Can you work these out from the model? Positions are in its coordinate system, mm. Face numbers are marked on the shaded views. A direction names the side the tool comes from. Give positions to 0.01 mm unless a question says otherwise; leave off trailing zeros. Order: outer loops, then holes, each group sorted by start corner. A loop starts at its lowest first (then second) coordinate and runs counter-clockwise, first axis right, second up. Notation, with made-up numbers: M -21.5,54.25 L -14.5,54.25 A23 cw -14.5,73.25 Z; hole C 45.25,-16 d4. An arc over 180 degrees is marked long. Write each question's results on one line, items separated by ' | '.
from build123d import *

# Parameters (mm, degrees)
ESQUISSE2_W                  = 56.5
ESQUISSE2_H                  = 38
ESQUISSE2_R                  = 3.05
ESQUISSE2_W_2                = 6
SOCLESYRINGE_DEPTH           = 12
ESQUISSE2_2_R                = 3.05
BOSS_EXTRU_2_DEPTH           = 3
ESQUISSE2_4_W                = 6
ESQUISSE2_4_H                = 38
BOSS_EXTRU_4_DEPTH           = 14
ESQUISSE3_W                  = 68.5
ESQUISSE3_H                  = 20
BOSS_EXTRU_3_DEPTH           = 12
ESQUISSE4_W                  = 11
ESQUISSE4_H                  = 5.5
ENL_V_MAT_EXTRU_1_DEPTH      = 10
CONG_1_R                     = 2.7
ESQUISSE6_W                  = 68.5
ESQUISSE6_H                  = 25
BOSS_EXTRU_5_DEPTH           = 15.5
BOSS_EXTRU_6_DEPTH           = 3.6
ENL_V_MAT_EXTRU_3_DEPTH      = 80.515611675
CONG_2_R                     = 1
ENL_V_MAT_EXTRU_2_DEPTH      = 76.059126694
ENL_V_MAT_EXTRU_2_DEPTH_BACK = 76.059126694
ESQUISSE5_R                  = 2.5
ESQUISSE9_R                  = 5.5
ENL_V_MAT_EXTRU_4_DEPTH      = 24


with BuildPart() as part:
    # Esquisse2 → SocleSyringe (new body)
    # profile 1 of 3: a face of its own
    with BuildSketch(Plane.XY):
        Rectangle(ESQUISSE2_W, ESQUISSE2_H)
        with Locations((-21.5, 9)):
            Circle(ESQUISSE2_R, mode=Mode.SUBTRACT)
        with Locations((21.5, 9)):
            Circle(ESQUISSE2_R, mode=Mode.SUBTRACT)
    # profile 2 of 3: a face of its own
    with BuildSketch(Plane.XY):
        with Locations((-31.25, 0)):
            Rectangle(ESQUISSE2_W_2, ESQUISSE2_H)
    # profile 3 of 3: a face of its own
    with BuildSketch(Plane.XY):
        with Locations((31.25, 0)):
            Rectangle(ESQUISSE2_W_2, ESQUISSE2_H)
    extrude(amount=SOCLESYRINGE_DEPTH)

    # Esquisse2<2> → Boss.-Extru.2 (add)
    with BuildSketch(Plane.XY):
        with Locations((-21.5, 9)):
            Circle(ESQUISSE2_2_R)
        with Locations((21.5, 9)):
            Circle(ESQUISSE2_2_R)
    extrude(amount=BOSS_EXTRU_2_DEPTH)

    # Esquisse2<4> → Boss.-Extru.4 (add)
    with BuildSketch(Plane.XY):
        with Locations((-31.25, 0)):
            Rectangle(ESQUISSE2_4_W, ESQUISSE2_4_H)
        with Locations((31.25, 0)):
            Rectangle(ESQUISSE2_4_W, ESQUISSE2_4_H)
    extrude(amount=BOSS_EXTRU_4_DEPTH)

    # Esquisse3 → Boss.-Extru.3 (add)
    with BuildSketch(Plane.XY):
        with Locations((0, 29)):
            Rectangle(ESQUISSE3_W, ESQUISSE3_H)
    extrude(amount=BOSS_EXTRU_3_DEPTH)

    # Esquisse4 → Enlèv. mat.-Extru.1 (cut)
    with BuildSketch(Plane.XY.offset(12)):
        with Locations((-23.75, 34)):
            Rectangle(ESQUISSE4_W, ESQUISSE4_H)
        with Locations((23.75, 34)):
            Rectangle(ESQUISSE4_W, ESQUISSE4_H)
        with Locations((23.75, 24)):
            Rectangle(ESQUISSE4_W, ESQUISSE4_H)
        with Locations((-23.75, 24)):
            Rectangle(ESQUISSE4_W, ESQUISSE4_H)
        with Locations((0, 34)):
            Rectangle(ESQUISSE4_W, ESQUISSE4_H)
        with Locations((0, 24)):
            Rectangle(ESQUISSE4_W, ESQUISSE4_H)
    extrude(amount=-ENL_V_MAT_EXTRU_1_DEPTH, mode=Mode.SUBTRACT)

    # Congé1
    cong_1_edges = [part.edges().sort_by_distance(p)[0] for p in [
        (23.75, 36.75, 2),
        (23.75, 31.25, 2),
        (23.75, 26.75, 2),
        (23.75, 21.25, 2),
        (-23.75, 21.25, 2),
        (-23.75, 26.75, 2),
        (0, 31.25, 2),
        (0, 36.75, 2),
        (0, 21.25, 2),
        (0, 26.75, 2),
        (-23.75, 31.25, 2),
        (-23.75, 36.75, 2),
    ]]
    fillet(cong_1_edges, radius=CONG_1_R)

    # Esquisse6 → Boss.-Extru.5 (add)
    with BuildSketch(Plane.XY):
        with Locations((0, 51.5)):
            Rectangle(ESQUISSE6_W, ESQUISSE6_H)
    extrude(amount=BOSS_EXTRU_5_DEPTH)

    # Esquisse7 → Boss.-Extru.6 (add)
    with BuildSketch(Plane.XY.offset(15.5)):
        Polygon((-34.25, 39), (-8.9, 39), (-8.9, 58.1), (0, 58.1), (0, 64), (-34.25, 64), align=None)
        Polygon((8.4, 58.1), (8.4, 39), (34.25, 39), (34.25, 64), (0, 64), (0, 58.1), align=None)
    extrude(amount=BOSS_EXTRU_6_DEPTH)

    # Esquisse8 → Enlèv. mat.-Extru.3 (cut, through all)
    with BuildSketch(Plane(origin=(-8.9, 0, 0), x_dir=(0, 0, -1), z_dir=(1, 0, 0))):
        with BuildLine():
            Line((-19.1, 51.05), (-19.1, 46.05))
            ThreePointArc((-19.1, 46.05), (-16.6, 48.55), (-19.1, 51.05))
        make_face()
    extrude(amount=-ENL_V_MAT_EXTRU_3_DEPTH, mode=Mode.SUBTRACT)

    # Congé2
    cong_2_edges = [part.edges().sort_by_distance(p)[0] for p in [
        (-8.9, 48.55, 15.5),
        (8.4, 48.55, 15.5),
    ]]
    fillet(cong_2_edges, radius=CONG_2_R)

    # Esquisse5 → Enlèv. mat.-Extru.2 (cut, two sides: drawn at the far end of the back side and taken through both)
    with BuildSketch(Plane(origin=(0, 0, 0), x_dir=(1, 0, 0), z_dir=(0, 1, 0)).offset(-ENL_V_MAT_EXTRU_2_DEPTH_BACK)):
        with Locations(Location((23.75, -7.6, 0), (0, 0, 270))):
            Circle(ESQUISSE5_R)
        with Locations((-23.75, -7.6)):
            Circle(ESQUISSE5_R)
        with Locations(Location((0, -7.6, 0), (0, 0, 90))):
            Circle(ESQUISSE5_R)
    extrude(amount=ENL_V_MAT_EXTRU_2_DEPTH + ENL_V_MAT_EXTRU_2_DEPTH_BACK, mode=Mode.SUBTRACT)

    # Esquisse9 → Enlèv. mat.-Extru.4 (cut)
    with BuildSketch(Plane(origin=(0, 64, 0), x_dir=(1, 0, 0), z_dir=(0, 1, 0))):
        with Locations(Location((-23.75, -7.6, 0), (0, 0, 270))):
            Circle(ESQUISSE9_R)
        with Locations(Location((0, -7.6, 0), (0, 0, 270))):
            Circle(ESQUISSE9_R)
        with Locations(Location((23.75, -7.6, 0), (0, 0, 270))):
            Circle(ESQUISSE9_R)
    extrude(amount=-ENL_V_MAT_EXTRU_4_DEPTH, mode=Mode.SUBTRACT)


solid = part.part
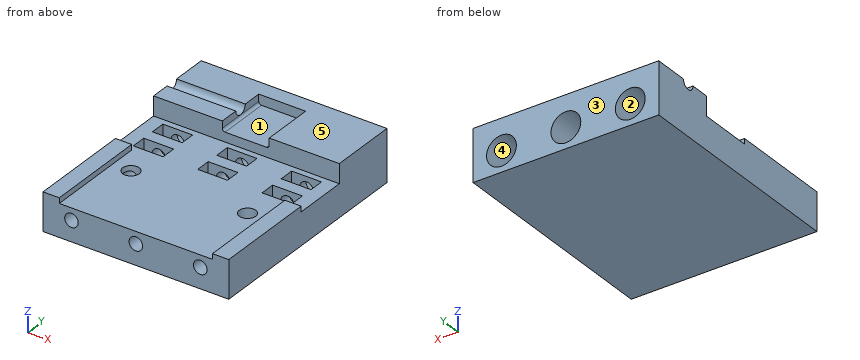
(1) Imagine slicing it at A-A, the plane y = 48.55. Write out the boundary of the cut face in (x, z).
Data:
outline: M -34.25,0 L 34.25,0 L 34.25,19.1 L 8.4,19.1 L 8.4,16.5 A1 cw 7.4,15.5 L -7.9,15.5 A1 cw -8.9,16.5 L -8.9,16.6 L -34.25,16.6 Z; hole C -23.75,7.6 d11; hole C 0,7.6 d11; hole C 23.75,7.6 d11
(2) We'd pull the mould along Z, two halves only. Please class the marked faces 1, 2 and 3: +Z half, -Z half, draft (parallel to the pull), parting line (faces both ways), or undercut.
Data:
face 1: +Z half | face 2: undercut | face 3: draft
(3) Imagine slicing it at C-C, the plane x = 13. Write out the boundary of the cut face in (y, z).
Data:
outline: M -19,0 L 64,0 L 64,19.1 L 39,19.1 L 39,12 L -19,12 Z
(4) For the marked faces 4 and 5, which set-ups out of +Z, -Z, +X, -X, +Y, -Y let a thin tool reach every point of the face, with its end or its side?
Data:
face 4: +Y | face 5: +Z, +X, -X, +Y, -Y
(5) Imagine slicing it at B-B, the plane y = 9. Write out the boundary of the cut face in (x, z), plus the area to 3 significant figures.
Data:
outline: M -34.25,0 L 34.25,0 L 34.25,14 L 28.25,14 L 28.25,12 L 24.55,12 L 24.55,9.97 A2.5 cw 24.55,5.23 L 24.55,3 L 18.45,3 L 18.45,12 L -18.45,12 L -18.45,3 L -24.55,3 L -24.55,5.23 A2.5 cw -24.55,9.97 L -24.55,12 L -28.25,12 L -28.25,14 L -34.25,14 Z; hole C 0,7.6 d5 | area: 705 mm2
(6) I need wall thicknesses on L1, parallel to X at y = 45, z = 8; L2, parallel to Y at x = 1.5, z = 11; L3, parallel to X at y = 39, z = 7.75. Which ranges of each line are inside material? Lowest first, please. Write a range as from..to.
Data:
L1: x = -34.25..-29.24, -18.26..-5.49, 5.49..18.26, 29.24..34.25 | L2: y = -19..21.25, 26.75..31.25, 36.75..40 | L3: x = -34.25..-26.25, -21.25..-2.5, 2.5..21.25, 26.25..34.25
(7) Imagine slicing it at D-D, the plane y = 18. Write out the boundary of the cut face in (x, z).
Data:
outline: M -34.25,0 L 34.25,0 L 34.25,14 L 28.25,14 L 28.25,12 L -28.25,12 L -28.25,14 L -34.25,14 Z; hole C -23.75,7.6 d5; hole C 0,7.6 d5; hole C 23.75,7.6 d5
(8) Will these pins go through, and if not, where does the flat tip stop? P1, Ø12, axis at x = -19.5, y = 1.5, coming from the +Z side; P2, Ø6.5, axis at x = -23.75, z = 7.6, coming from the +Y side; P3, Ø3, axis at x = 32.5, y = 6.5, coming from the +Z side; P4, Ø12, axis at x = 1.5, y = 24, coming from the -Z side.
Data:
P1: stops at z = 12 | P2: stops at y = 40 | P3: stops at z = 14 | P4: stops at z = 0
